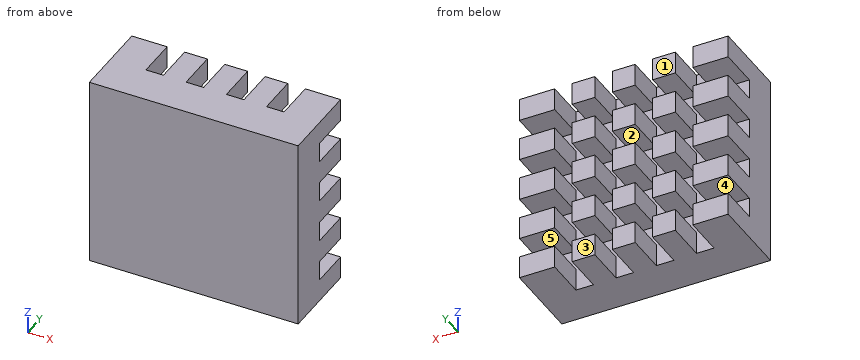
from build123d import *

# Parameters (mm, degrees)
SKETCH1_W           = 13
SKETCH1_H           = 12
BOSS_EXTRUDE1_DEPTH = 5
SKETCH2_W           = 1.41
SKETCH2_H           = 1.4
SKETCH2_H_2         = 1.44
SKETCH2_W_2         = 1.42
CUT_EXTRUDE1_DEPTH  = 2.5


with BuildPart() as part:
    # Sketch1 → Boss-Extrude1 (new body)
    with BuildSketch(Plane(origin=(0, 0, 0), x_dir=(1, 0, 0), z_dir=(0, 1, 0))):
        Rectangle(SKETCH1_W, SKETCH1_H)
    extrude(amount=BOSS_EXTRUDE1_DEPTH)

    # Sketch2 → Cut-Extrude1 (cut)
    with BuildSketch(Plane(origin=(0, 5, 0), x_dir=(1, 0, 0), z_dir=(0, 1, 0))):
        Polygon((-1.8, 6), (-0.71, 6), (-0.71, 4.6), (0.71, 4.6), (0.71, 6), (1.8, 6), (1.8, 4.6), (3.21, 4.6), (3.21, 6), (4.3, 6), (4.3, 4.6), (6.5, 4.6), (6.5, 3.36), (4.3, 3.36), (4.3, 1.96), (6.5, 1.96), (6.5, 0.72), (4.3, 0.72), (4.3, -0.72), (6.5, -0.72), (6.5, -1.96), (4.3, -1.96), (4.3, -3.36), (6.5, -3.36), (6.5, -4.6), (4.3, -4.6), (4.3, -6), (3.21, -6), (3.21, -4.6), (1.8, -4.6), (1.8, -6), (0.71, -6), (0.71, -4.6), (-0.71, -4.6), (-0.71, -6), (-1.8, -6), (-1.8, -4.6), (-3.21, -4.6), (-3.21, -6), (-4.3, -6), (-4.3, -4.6), (-6.5, -4.6), (-6.5, -3.36), (-4.3, -3.36), (-4.3, -1.96), (-6.5, -1.96), (-6.5, -0.72), (-4.3, -0.72), (-4.3, 0.72), (-6.5, 0.72), (-6.5, 1.96), (-4.3, 1.96), (-4.3, 3.36), (-6.5, 3.36), (-6.5, 4.6), (-4.3, 4.6), (-4.3, 6), (-3.21, 6), (-3.21, 4.6), (-1.8, 4.6), align=None)
        with Locations((-2.505, -2.66)):
            Rectangle(SKETCH2_W, SKETCH2_H, mode=Mode.SUBTRACT)
        with Locations((-2.505, 0)):
            Rectangle(SKETCH2_W, SKETCH2_H_2, mode=Mode.SUBTRACT)
        with Locations((-2.505, 2.66)):
            Rectangle(SKETCH2_W, SKETCH2_H, mode=Mode.SUBTRACT)
        with Locations((2.505, -2.66)):
            Rectangle(SKETCH2_W, SKETCH2_H, mode=Mode.SUBTRACT)
        with Locations((0, -2.66)):
            Rectangle(SKETCH2_W_2, SKETCH2_H, mode=Mode.SUBTRACT)
        Rectangle(SKETCH2_W_2, SKETCH2_H_2, mode=Mode.SUBTRACT)
        with Locations((0, 2.66)):
            Rectangle(SKETCH2_W_2, SKETCH2_H, mode=Mode.SUBTRACT)
        with Locations((2.505, 2.66)):
            Rectangle(SKETCH2_W, SKETCH2_H, mode=Mode.SUBTRACT)
        with Locations((2.505, 0)):
            Rectangle(SKETCH2_W, SKETCH2_H_2, mode=Mode.SUBTRACT)
    extrude(amount=-CUT_EXTRUDE1_DEPTH, mode=Mode.SUBTRACT)


solid = part.part
Here's how the part is built. I have some questions about the finished solid (model axes, mm). Face numbers are marked on the shaded views. A direction names the side the tool comes from. Coordinates: 2 decimals unless noted, no trailing zeros. Order: outer loops, then holes, each group sorted by start corner. A loop starts at its lowest first (then second) coordinate and runs counter-clockwise, first axis right, second up. Notation, with made-up numbers: M -5,36 L 23,36 A21 cw 23,70 Z; hole C 76.5,29.25 d6. An arc over 180 degrees is marked long. Answer as CSV lines item,"result". Start each with the question number.
1. I need wall thicknesses on line 1 (Z direction, x = 4.75, y = 3.85); line 2 (Y direction, x = 3.5, z = 4.25). Which ranges of each line are inside material? Lowest first, please. Write a range as [from, to].
2. I want a section at D-D, the plane z = -1.75. Write out the boundary of the cut face in (x, y).
3. I want a section at C-C, the plane z = 0.5. Write out the boundary of the cut face in (x, y), and give its area (3 significant figures).
4. I want a section at B-B, the plane y = 4.65. Count the separate pieces of the cut face and the enclosed holes in it, and give its area (3 significant figures).
5. I want a section at A-A, the plane x = -0.25. Write out the boundary of the cut face in (y, z), and give its area (3 significant figures).
6. We'd pull the mould along Z, two halves only. Please class the marked faces 3, 4 and 5: released by +Z, released by -Z, zero draft, split by the parting line, or undercut.
7. On a 3-axis mill with a long thin cutter (end or side, diameter ignored), from which of +Z, -Z, +X, -X, +Y, -Y can I reach the whole of each face in a straight line? I mean the marked faces 1 and 2. Say none if no direction works.
Recorded:
1,line 1,"z = [-6, -4.6], [-3.36, -1.96], [-0.72, 0.72], [1.96, 3.36], [4.6, 6]"
1,line 2,"y = [0, 2.5]"
2,outline,"M -6.5,0 L 6.5,0 L 6.5,2.5 L -6.5,2.5 Z"
3,outline,"M -6.5,0 L 6.5,0 L 6.5,5 L 4.3,5 L 4.3,2.5 L 3.21,2.5 L 3.21,5 L 1.8,5 L 1.8,2.5 L 0.71,2.5 L 0.71,5 L -0.71,5 L -0.71,2.5 L -1.8,2.5 L -1.8,5 L -3.21,5 L -3.21,2.5 L -4.3,2.5 L -4.3,5 L -6.5,5 Z"
3,area,"54.1 mm2"
4,separate pieces,"25"
4,enclosed holes,"0"
4,area,"60.8 mm2"
5,outline,"M 0,-6 L 5,-6 L 5,-4.6 L 2.5,-4.6 L 2.5,-3.36 L 5,-3.36 L 5,-1.96 L 2.5,-1.96 L 2.5,-0.72 L 5,-0.72 L 5,0.72 L 2.5,0.72 L 2.5,1.96 L 5,1.96 L 5,3.36 L 2.5,3.36 L 2.5,4.6 L 5,4.6 L 5,6 L 0,6 Z"
5,area,"47.6 mm2"
6,face 3,"zero draft"
6,face 4,"undercut"
6,face 5,"undercut"
7,face 1,"+Z, -Z, +X, -X, +Y"
7,face 2,"+X, -X, +Y"
